from build123d import *

# Parameters (mm, degrees)
SKETCH1_W           = 140
SKETCH1_H           = 75
BOSS_EXTRUDE1_DEPTH = 35
SHELL1_T            = -2.5
FILLET1_R           = 2


with BuildPart() as part:
    # Sketch1 → Boss-Extrude1 (new body)
    with BuildSketch(Plane.XY):
        Rectangle(SKETCH1_W, SKETCH1_H)
    extrude(amount=BOSS_EXTRUDE1_DEPTH)

    # Shell1
    shell1_openings = [part.faces().sort_by_distance(p)[0] for p in [
        (0, 0, 0),
    ]]
    offset(amount=SHELL1_T, openings=shell1_openings, kind=Kind.INTERSECTION)

    # Fillet1
    fillet1_edges = [part.edges().sort_by_distance(p)[0] for p in [
        (70, -37.5, 17.5),
        (-70, -37.5, 17.5),
        (-70, 37.5, 17.5),
        (70, 37.5, 17.5),
    ]]
    fillet(fillet1_edges, radius=FILLET1_R)


solid = part.part
Check sheet for the modelled part. Datum: model origin and axes. Units: mm. A direction names the side the tool comes from. Give positions to 0.01 mm unless a question says otherwise; leave off trailing zeros. Write each loop counter-clockwise with the first axis right and the second up, starting at its lowest first coordinate (ties: lowest second). Pieces come first, ordered by that corner, then holes. Notation, with made-up numbers: (8, -35) -> (65, -35) arc R22 cw to (65, -8) -> close; hole circle Ø3 at (30, 12). An arc over 180 degrees is marked (long way). One line per item, written item: value. Start each with the question number.
Item 1: Tool access check on faces 1 (the flat face through (-1, -37.5, 17)), 2 (the flat face through (-1, -35, 16)). Record the directions out of +Z, -Z, +X, -X, +Y, -Y that give a thin tool (end or side, any length) a straight path to the whole face; none if there is none.
Item 2: Section check C-C on y = -30. Record the cut outline in (x, z), then the cut area to 4 significant figures.
Item 3: Section check A-A on x = -37. Record the cut outline in (y, z), then the cut area to 3 significant figures.
Item 4: Draft check along X on faces 3 (the flat face through (-1, 35, 16)), 4 (the flat face through (-70, 0, 17)), 5 (the flat face through (-1, 1, 35)). Enter one of: +X half, -X half, draft (parallel to the pull), parting line (faces both ways), or undercut.
Item 5: Section check B-B on z = 2.5. Record the cut outline in (x, y).
Item 6: Material ranges on probe 1 along X at (y, z) = (-8, 18); probe 2 along Y at (x, z) = (38.5, 31.5); probe 3 along Z at (x, y) = (30, 4), recorded low to high. Write a range as from..to.
Item 7: Gauge pin test, flat end, axial feed: pin 1 (3 mm diameter, centred on x = -47.5, y = -29, fed in from -Z). Record the tip position at first contact, or that the pin passes through.
Results list:
1. face 1: +Z, -Z, +X, -X, -Y
1. face 2: -Z
2. outline: (-70, 0) -> (-67.5, 0) -> (-67.5, 32.5) -> (67.5, 32.5) -> (67.5, 0) -> (70, 0) -> (70, 35) -> (-70, 35) -> close
2. area: 512.5 mm²
3. outline: (-37.5, 0) -> (-35, 0) -> (-35, 32.5) -> (35, 32.5) -> (35, 0) -> (37.5, 0) -> (37.5, 35) -> (-37.5, 35) -> close
3. area: 350 mm²
4. face 3: undercut
4. face 4: -X half
4. face 5: draft
5. outline: (-70, -35.5) arc R2 ccw to (-68, -37.5) -> (68, -37.5) arc R2 ccw to (70, -35.5) -> (70, 35.5) arc R2 ccw to (68, 37.5) -> (-68, 37.5) arc R2 ccw to (-70, 35.5) -> close; hole (-67.5, -35) -> (67.5, -35) -> (67.5, 35) -> (-67.5, 35) -> close
6. probe 1: -70..-67.5, 67.5..70
6. probe 2: -37.5..-35, 35..37.5
6. probe 3: 32.5..35
7. pin 1: z = 32.5
